Source: CAD feature listing. Evaluate the final solid. Frame: model axes, mm. Face numbers are marked on the shaded views. A direction names the side the tool comes from. Round coordinates to 2 decimals unless told otherwise and drop trailing zeros. Write each loop counter-clockwise with the first axis right and the second up, starting at its lowest first coordinate (ties: lowest second). Pieces come first, ordered by that corner, then holes. Notation, with made-up numbers: (-33.75, 28.5) -> (-1.75, 28.5) arc R29 cw to (-1.75, 65.5) -> close; hole circle Ø10 at (47.25, 71.5). An arc over 180 degrees is marked (long way). Put each result on its own line as item: value.
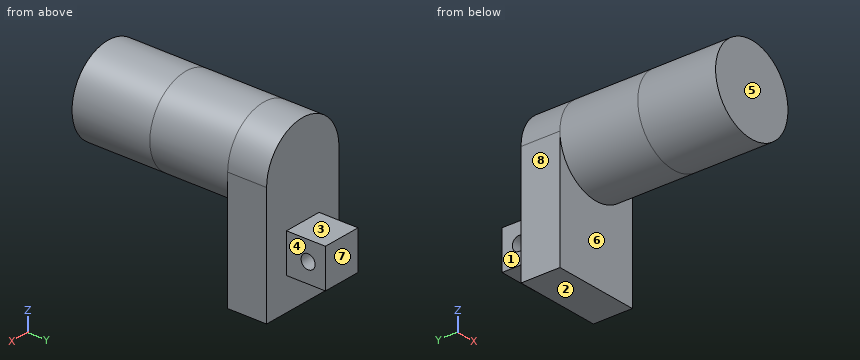
Autodesk Fusion 360 part; units mm, degrees
sketch "Sketch1" plane through (0, 0, 0) normal (0, 0, 1) x (1, 0, 0)
sketch "Sketch2" plane through (0, 0, 0) normal (1, 0, 0) x (0, 1, 0)
  line L0 (36, -20) -> (-36, -20)
  line L1 (-36, -20) -> (-36, 20)
  line L2 (-36, 20) -> (36, 20)
  line L3 (36, 20) -> (36, -20)
  line L4 (36, -20) -> (-36, 20) construction
  line L5 (-36, -20) -> (36, 20) construction
  dimension "d1" = 72
  dimension "d2" = 40
sketch "Sketch3" plane through (0, 0, 0) normal (0, 1, 0) x (1, 0, 0)
  circle A0 centre (0, 0) radius 20
  dimension "d3" = 40
extrude "Extrude1" add sketch "Sketch3" along normal mid plane 72
sketch "Sketch4" plane through (0, 0, 0) normal (0, 1, 0) x (1, 0, 0)
sketch "Sketch5" plane through (0, 36, 0) normal (0, 1, 0) x (-1, 0, 0)
  circle A0 centre (0, 0) radius 20
  circle A1 centre (0, 0) radius 20
  line L0 (0, 20) -> (0, -55) construction
  line L1 (20, 0) -> (20, -55)
  line L2 (20, -55) -> (-20, -55)
  line L3 (-20, -55) -> (-20, 0)
  line L4 (0, -55) -> (0, -31) construction
  line L5 (9, -40) -> (-9, -40)
  line L6 (-9, -40) -> (-9, -22)
  line L7 (-9, -22) -> (9, -22)
  line L8 (9, -22) -> (9, -40)
  line L9 (9, -40) -> (-9, -22) construction
  line L10 (-9, -40) -> (9, -22) construction
  line L11 (20, -19.9504) -> (-20, -19.9504)
  line L12 (-20, -19.9504) -> (-20, -49.9504)
  line L13 (-20, -49.9504) -> (20, -49.9504)
  line L14 (20, -49.9504) -> (20, -19.9504)
  point P0 (0, -31)
  dimension "d6" = 75
  dimension "d11" = 24
  dimension "d12" = 18
  dimension "d21" = 30
extrude "Extrude2" add sketch "Sketch5" along normal blind 18 contours A0 A1 L11 | A0 A1 L1 L11 | A0 A1 L3 L11 | A0 A1 L1 L3 L11 L12 L13 L14 | A0 A1 L11 | L1 L2 L3 L13 | L5 L6 L7 L8
extrude "Extrude4" add sketch "Sketch5" along normal blind 36 contours L5 L6 L7 L8
sketch "Sketch6" plane through (0, 0, 0) normal (1, 0, 0) x (0, 1, 0)
  line L0 (54, -22) -> (72, -40) construction
  line L1 (72, -40) -> (72, -22) construction
  line L2 (72, -22) -> (54, -40) construction
  line L3 (54, -40) -> (63, -31) construction
  line L4 (54, -31) -> (64, -31) construction
  circle A0 centre (64, -31) radius 3.25
  dimension "d17" = 10
  dimension "d18" = 6.5
extrude "Extrude5" cut sketch "Sketch6" along normal mid plane 64
extrude "Extrude6" [suppressed]
extrude "Extrude3" [suppressed]
Q1. Material intervals for line 1 (Z direction, x = -5, y = 64); line 2 (Y direction, x = 4.5, z = -31); line 3 (Y direction, x = -6, z = -36.5), sorted ascending. Write a range as [from, to].
Ans:
line 1: z = [-40, -34.25], [-27.75, -22]
line 2: y = [36, 60.75], [67.25, 72]
line 3: y = [36, 72]
Q2. Draft query along Y for the marked faces 6, 7 and 8. Return one class per face: +Y half, -Y half, draft (parallel to the pull), parting line (faces both ways), or undercut.
Ans:
face 6: -Y half
face 7: +Y half
face 8: draft
Q3. Cut plane A-A on y = 64. Output: boundary loops of the cut face in (x, z).
Ans:
outline: (-9, -40) -> (9, -40) -> (9, -34.25) -> (-9, -34.25) -> close; (-9, -27.75) -> (9, -27.75) -> (9, -22) -> (-9, -22) -> close
Q4. Cut plane C-C on x = -5. Output: boundary loops of the cut face in (y, z).
Ans:
outline: (-36, -19.36) -> (36, -19.36) -> (36, -55) -> (54, -55) -> (54, -40) -> (72, -40) -> (72, -22) -> (54, -22) -> (54, 19.36) -> (-36, 19.36) -> close; hole circle Ø6.5 at (64, -31)
Q5. Cut plane D-D on z = -13. Output: boundary loops of the cut face in (x, y), and give its area (3 significant figures).
Ans:
outline: (-20, 36) -> (-15.2, 36) -> (-15.2, -36) -> (15.2, -36) -> (15.2, 36) -> (20, 36) -> (20, 54) -> (-20, 54) -> close
area: 2,910 mm^2
Q6. Reachability of the marked faces 1, 2, 3, 4 and 5 from +Z, -Z, +X, -X, +Y, -Y: full face, straight path, thin tool, end or side. Return the list, or none.
Ans:
face 1: +Z, -Z, -X, +Y
face 2: -Z, +X, -X, +Y, -Y
face 3: +Z, +X, -X, +Y
face 4: +Z, -Z, +X, +Y
face 5: +Z, -Z, +X, -X, -Y
Q7. Cut plane B-B on z = -31. Output: boundary loops of the cut face in (x, y), and give its area (3 significant figures).
Ans:
outline: (-20, 36) -> (20, 36) -> (20, 54) -> (9, 54) -> (9, 60.75) -> (-9, 60.75) -> (-9, 54) -> (-20, 54) -> close; (-9, 67.25) -> (9, 67.25) -> (9, 72) -> (-9, 72) -> close
area: 927 mm^2
Q8. Pin query (flat end, axial travel): pin 1 (2 mm diameter, centred on x = -13, y = 6.5, fed in from -Z); pin 2 (2 mm diameter, centred on x = 2.5, z = -47, fed in from +Y); pin 3 (20 mm diameter, centred on x = -1.5, y = 64.5, fed in from +Z); pin 4 (14.5 mm diameter, centred on x = -2.5, y = 59.5, fed in from -Z). Return the tip coordinate at first contact, or that it passes through.
Ans:
pin 1: stops at z = -16
pin 2: stops at y = 54
pin 3: stops at z = -22
pin 4: stops at z = -55
